Can you work these out from the model? Positions are in its coordinate system, mm. A direction names the side the tool comes from. Round coordinates to 2 decimals unless told otherwise and drop trailing zeros. Order: outer loops, then holes, each group sorted by start corner. A loop starts at its lowest first (then second) coordinate and runs counter-clockwise, first axis right, second up.
Q1. If we section it at A-A (y = -55): Please give me the cut outline in (x, z).
Q2. If I drill on line 1 (Y direction, x = 239, z = 0.9); line 2 (Y direction, x = 211, z = 1.35); line 3 (X direction, y = -60, z = 0.1), over which ranges is the centre line in solid material (lowest first)?
Q3. If we section it at D-D (x = 248): Please give me the cut outline in (y, z).
Q4. We'd pull the mould along X, two halves only. Please class faces 1 (the face through (242, -22, 1.524)), 2 (the face through (246.792, -66.153, 0.751)), 3 (the face through (264.77, -64.07, 0.75)), 4 (the face through (197.759, -67.615, 0.751)): pulls with the +X half, pulls with the -X half, needs draft (parallel to the pull), parting line crosses it, or undercut.
Q5. If we section it at B-B (x = 218): Please give me the cut outline in (y, z).
Q6. If we section it at C-C (x = 209.5): Please give me the cut outline in (y, z), plus the area to 3 significant figures.
Q7. For faces 5 (the face through (253.97, -73.11, 0.75)), 6 (the face through (200.975, -79.276, 0.751)), 7 (the face through (221.86, -72.69, 0.75)), which set-ups out of +Z, -Z, +X, -X, +Y, -Y let a thin tool reach every point of the face, with its end or its side?
Q8. Will these pins go through, and if not, where does the flat tip stop? P1, Ø0.5, axis at y = -1, z = 1, coming from the -X side; P2, Ø0.8, axis at y = -76, z = 0.5, coming from the +X side.
from build123d import *

# Parameters (mm, degrees)
BOSS_EXTRUDE1_DEPTH = 1.524


with BuildPart() as part:
    # Sketch1 → Boss-Extrude1 (new body)
    with BuildSketch(Plane.XY):
        with BuildLine():
            Line((211.523731391, 0), (211.523731391, -2.54))
            Line((211.523731391, -2.54), (202.922883793, -2.527561419))
            ThreePointArc((202.922883793, -2.527561419), (213.740389033, -12.255488314), (228.152940708, -14.237743463))
            ThreePointArc((228.152940708, -14.237743463), (229.717824369, -14.48375454), (230.832595731, -15.609217614))
            ThreePointArc((230.832595731, -15.609217614), (237.419060845, -23.79840587), (246.808881255, -28.518109213))
            ThreePointArc((246.808881255, -28.518109213), (240.118021125, -46.587905071), (250.249852394, -62.977875381))
            ThreePointArc((250.249852394, -62.977875381), (246.752221114, -66.207121421), (244.693512184, -70.499343702))
            ThreePointArc((244.693512184, -70.499343702), (243.933055031, -71.742181277), (242.614733859, -72.362640469))
            ThreePointArc((242.614733859, -72.362640469), (221.562461662, -72.654811524), (201.196110579, -67.316715223))
            ThreePointArc((201.196110579, -67.316715223), (197.716188185, -67.641087637), (195.87163248, -70.609705427))
            ThreePointArc((195.87163248, -70.609705427), (189.064028536, -74.973109583), (185.80791446, -82.374493805))
            ThreePointArc((185.80791446, -82.374493805), (201.196110579, -79.270242267), (216.71630717, -81.627455706))
            ThreePointArc((216.71630717, -81.627455706), (222.189556026, -82.374432464), (227.713542567, -82.374493805))
            ThreePointArc((227.713542567, -82.374493805), (239.353709896, -81.313035156), (250.993877225, -82.374493805))
            ThreePointArc((250.993877225, -82.374493805), (253.605845534, -80.999769877), (252.438715023, -78.288672185))
            ThreePointArc((252.438715023, -78.288672185), (251.512482649, -77.574775104), (250.632502883, -76.804586124))
            Line((250.632502883, -76.804586124), (220.3898048, -76.789947691))
            Line((220.3898048, -76.789947691), (220.3898048, -75.265947691))
            Line((220.3898048, -75.265947691), (250.581391322, -75.229531899))
            ThreePointArc((250.581391322, -75.229531899), (254.019892125, -73.080630034), (257.482403047, -70.97063356))
            Line((257.482403047, -70.97063356), (250.916170957, -37.690058187))
            Line((250.916170957, -37.690058187), (252.411347424, -37.395061012))
            Line((252.411347424, -37.395061012), (258.871697415, -70.138978964))
            ThreePointArc((258.871697415, -70.138978964), (260.416031898, -69.224443913), (261.964911432, -68.317627754))
            ThreePointArc((261.964911432, -68.317627754), (264.784241837, -63.996035266), (263.641101809, -58.964334117))
            ThreePointArc((263.641101809, -58.964334117), (257.882003246, -44.635324676), (262.978270283, -30.057403353))
            ThreePointArc((262.978270283, -30.057403353), (263.656491571, -28.633675993), (263.566043061, -27.059254582))
            ThreePointArc((263.566043061, -27.059254582), (262.588823269, -23.547314792), (261.873711132, -19.972780664))
            ThreePointArc((261.873711132, -19.972780664), (261.52305104, -19.036925788), (260.838506947, -18.308786906))
            ThreePointArc((260.838506947, -18.308786906), (256.845813142, -12.310330809), (257.874930037, -5.178430798))
            ThreePointArc((257.874930037, -5.178430798), (258.196394426, -3.928637169), (257.862228141, -2.682179643))
            ThreePointArc((257.862228141, -2.682179643), (241.665574941, 12.306611524), (219.801437593, 15.299091023))
            Line((219.801437593, 15.299091023), (203.553625304, 8.095778667))
            Line((203.553625304, 8.095778667), (202.1481549, 0.013558997))
            Line((202.1481549, 0.013558997), (211.523731391, 0))
        make_face()
    extrude(amount=BOSS_EXTRUDE1_DEPTH)


solid = part.part
Solution:
1. outline: (242.73, 0) - (254.33, 0) - (254.33, 1.52) - (242.73, 1.52) - close; (255.88, 0) - (260.75, 0) - (260.75, 1.52) - (255.88, 1.52) - close
2. line 1: y = -81.31 to -76.8, -75.24 to -72.82, -24.97 to 13.44
2. line 2: y = -80.11 to -70.62, -10.77 to -2.54, 0 to 11.4
2. line 3: x = 246.51 to 255.32, 256.87 to 264.25
3. outline: (-81.9, 0) - (-76.8, 0) - (-76.8, 1.52) - (-81.9, 1.52) - close; (-75.23, 0) - (-64.76, 0) - (-64.76, 1.52) - (-75.23, 1.52) - close; (-61.35, 0) - (8.49, 0) - (8.49, 1.52) - (-61.35, 1.52) - close
4. face 1: needs draft
4. face 2: undercut
4. face 3: pulls with the +X half
4. face 4: undercut
5. outline: (-81.87, 0) - (-72.14, 0) - (-72.14, 1.52) - (-81.87, 1.52) - close; (-13.78, 0) - (14.5, 0) - (14.5, 1.52) - (-13.78, 1.52) - close
6. outline: (-79.84, 0) - (-70.21, 0) - (-70.21, 1.52) - (-79.84, 1.52) - close; (-9.75, 0) - (-2.54, 0) - (-2.54, 1.52) - (-9.75, 1.52) - close; (0, 0) - (10.73, 0) - (10.73, 1.52) - (0, 1.52) - close
6. area: 42.0 mm2
7. face 5: +Z, -Z, +X
7. face 6: +Z, -Z, -Y
7. face 7: +Z, -Z
8. P1: stops at x = 211.52
8. P2: stops at x = 220.39
